Source: three-view drawing plus pictorial views. Frame: mm from the lowest corner of the part. Round coordinates to 2 decimals unless told otherwise and drop trailing zeros. Order: outer loops, then holes, each group sorted by start corner. A loop starts at its lowest first (then second) coordinate and runs counter-clockwise, first axis right, second up. Notation, with made-up numbers: (33, 84) - (48, 84) arc R4 ccw to (48, 88) - close; hole circle Ø10 at (11, 81). An arc over 180 degrees is marked (long way). Use one line per item in the form item = value. Start each with the question number.
Q1. Pin query (flat end, axial travel): pin 1 Ø22.5 at (x, y) = (47.5, 20) entering from +Z; pin 2 Ø1 at (y, z) = (36, 5) entering from -X. Return the tip coordinate at first contact, or that it passes through.
Q2. Ray query, line 1 (X direction, y = 16.5, z = 0.6); line 2 (Y direction, x = 47.5, z = 4.75); line 3 (Y direction, x = 10, z = 2). Return the intervals inside material, ascending. Write a range as [from, to].
Q3. Cut plane A-A, the plane x = 47.5. Return the cut outline in (y, z), and give its area (3 significant figures).
Q4. Cut plane C-C, the plane z = 1.75. Return the cut outline in (x, y).
Q5. Draft query along X for the marked faces 1, 2 and 3. Return one class per face: released by +X, released by -X, zero draft, split by the parting line, or undercut.
Q6. Cut plane B-B, the plane y = 20. Return the cut outline in (x, z), and give its area (3 significant figures).
Q7. Cut plane D-D, the plane y = 35. Return the cut outline in (x, z), and give its area (3 significant figures).
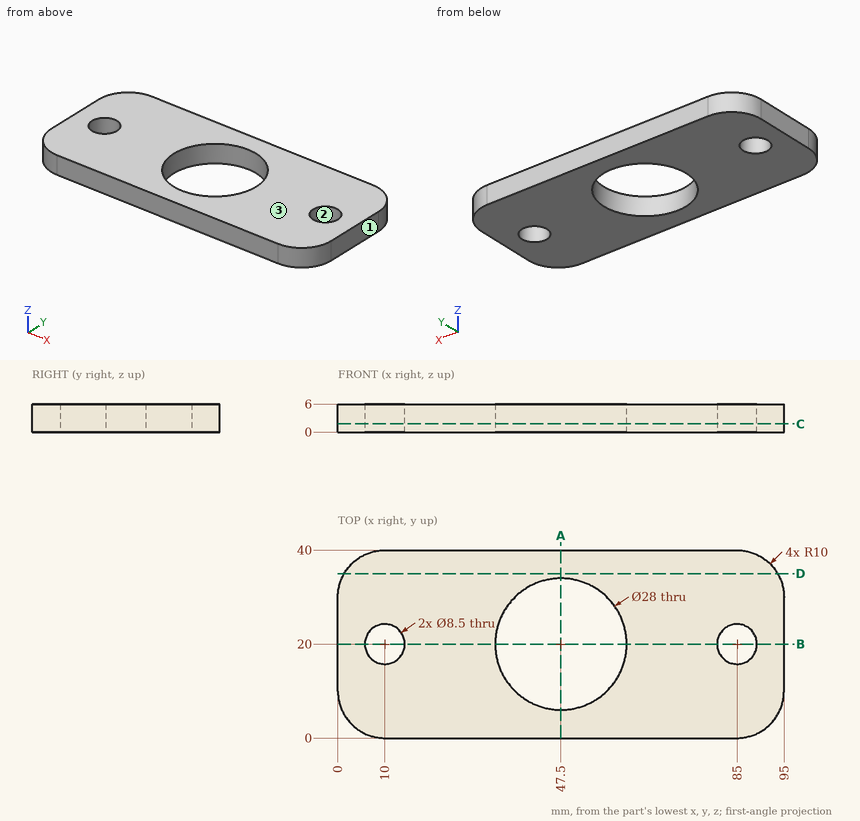
Completed:
q1.pin_1 = through
q1.pin_2 = 1.65
q2.line_1 = [0, 7.59], [12.41, 33.94], [61.06, 82.59], [87.41, 95]
q2.line_2 = [0, 6], [34, 40]
q2.line_3 = [0, 15.75], [24.25, 40]
q3.outline = (0, 0) - (6, 0) - (6, 6) - (0, 6) - close; (34, 0) - (40, 0) - (40, 6) - (34, 6) - close
q3.area = 72.0 mm2
q4.outline = (0, 10) arc R10 ccw to (10, 0) - (85, 0) arc R10 ccw to (95, 10) - (95, 30) arc R10 ccw to (85, 40) - (10, 40) arc R10 ccw to (0, 30) - close; hole circle Ø8.5 at (10, 20); hole circle Ø28 at (47.5, 20); hole circle Ø8.5 at (85, 20)
q5.face_1 = released by +X
q5.face_2 = undercut
q5.face_3 = zero draft
q6.outline = (0, 0) - (5.75, 0) - (5.75, 6) - (0, 6) - close; (14.25, 0) - (33.5, 0) - (33.5, 6) - (14.25, 6) - close; (61.5, 0) - (80.75, 0) - (80.75, 6) - (61.5, 6) - close; (89.25, 0) - (95, 0) - (95, 6) - (89.25, 6) - close
q6.area = 300 mm2
q7.outline = (1.34, 0) - (93.66, 0) - (93.66, 6) - (1.34, 6) - close
q7.area = 554 mm2
